Verification items for the finished model (mm, model axes). A direction names the side the tool comes from. Coordinates: 2 decimals unless noted, no trailing zeros. Write each loop counter-clockwise with the first axis right and the second up, starting at its lowest first coordinate (ties: lowest second). Pieces come first, ordered by that corner, then holes. Notation, with made-up numbers: (31.25, 73) -> (44.25, 73) arc R31 ccw to (44.25, 101) -> close; hole circle Ø6 at (87.5, 28). An arc over 180 degrees is marked (long way). Answer in a Markdown table with one row per item.
Autodesk Inventor part; units mm, degrees
ref_plane "Work Plane1" through (1.525, 0, 0) normal (0, 0, 1) x (1, 0, 0)
ref_plane "YZ Plane" through (0, 0, 0) normal (1, 0, 0) x (0, 1, 0)
ref_plane "XZ Plane" through (0, 0, 0) normal (0, 1, 0) x (-1, 0, 0)
sketch "Sketch1" plane through (0, 0, 0) normal (0, 0, 1) x (1, 0, 0)
  line L0 (0, 4) -> (55, 4)
  line L1 (55, 4) -> (55, 0)
  line L2 (55, 0) -> (0, 0)
  line L3 (-11, 0) -> (66, 0)
  line L4 (0, -0.8) -> (0, 4.8)
  line L5 (0, 4) -> (0, 0)
  dimension "d2" = 8
  dimension "d59" = 55
revolve "Body" add sketch "Sketch1" angle 360 about axis through (55, 0, 0) along (-1, 0, 0)
sketch "Sketch2" plane through (0, 0, 0) normal (-1, 0, 0) x (0, 0, 1)
  line L0 (0, 7.5056) -> (6.5, 3.7528)
  line L1 (6.5, 3.7528) -> (6.5, -3.7528)
  line L2 (6.5, -3.7528) -> (0, -7.5056)
  line L3 (0, -7.5056) -> (-6.5, -3.7528)
  line L4 (-6.5, -3.7528) -> (-6.5, 3.7528)
  line L5 (-6.5, 3.7528) -> (0, 7.5056)
  line L6 (-9.1, 0) -> (9.1, 0)
  line L7 (0, 10.5078) -> (0, -10.5078)
  point P0 (0, 0)
  point P1 (0, 0)
  dimension "d11" = 13
extrude "Head" add sketch "Sketch2" along normal blind 5.68
sketch "Sketch4" plane through (0, 0, 0) normal (0, 0, 1) x (1, 0, 0)
  line L0 (-4.9294, 7.8) -> (-5.68, 6.5)
  line L1 (-1.1, 0) -> (-0.234, 0)
  line L2 (-6.7692, 0) -> (0.8552, 0)
  line L3 (-5.68, 7.8) -> (-4.9294, 7.8)
  line L4 (-5.68, 6.5) -> (-5.68, 7.8)
  line L5 (0, 9.36) -> (0, -1.56)
  dimension "d65" = 13
  dimension "d67" = 30
  dimension "d68" = 15.6
  dimension "d69" = 5.68
revolve "Chamfer1" cut sketch "Sketch4" angle 360 about axis through (-1.1, 0, 0) along (1, 0, 0)
thread "Thread"
chamfer "Chamfer2" distance 0.7668 distance2 0.7669 1 edges at (55, -4, 0) measured on face at (55, -1.1806, 1.575)
fillet "Fillet" radius 0.1 1 edges at (0, -4, 0)
ref_plane "Work Plane1" through (1.525, 0, 0) normal (0, 0, 1) x (1, 0, 0)
equation "\"d2\" = GD"
equation "\"d59\" = NLG"
equation "\"d11\" = SW"
equation "\"d3\" = KOH"
equation "\"d15\" = GEL"
equation "\"d6\" = -0.5 * SPD + 0.5 * GD"
equation "\"d71\" = RR"
equation "\"d65\" = SW"
equation "\"d67\" = ANG1"
equation "\"d68\" = 1.2 * SW"
equation "\"d69\" = KOH"
equation "\"NLG\" = 55"
equation "\"GD\" = NND"
equation "\"BDM\" = NND"
equation "\"KOH\" = 5.68"
equation "\"GEL\" = 22"
equation "\"SW\" = 13"
equation "\"SW0\" = SW"
equation "\"SPD\" = NND - 1.2269 * PTC"
equation "\"SD2\" = NND"
equation "\"SD\" = 0"
equation "\"ANG1\" = 30deg"
equation "\"GAL\" = 0.61345 * PTC"
equation "\"GUL\" = 0.61345 * PTC"
equation "\"RR\" = 0.1"
equation "\"RR1\" = 0.4"
equation "\"GD1\" = THREADDIA - 1.2269 * PTC"
equation "\"THREADDIA\" = 8"
equation "\"TOA\" = 30deg"
equation "\"PTC\" = 1.25"
equation "\"KOH1\" = 3.7"
equation "\"NND\" = 8"
equation "\"E0\" = 1.155 * SW"
properties part number "ANSI B18.2.3.5M - M8 x 1.25 x 55" material "Steel, Mild"
1. Thickness scan on line 1 (X direction, y = 3.5, z = 5); line 2 (Y direction, x = -2.5, z = 1.75); line 3 (Z direction, x = 50.5, y = 0.25). Record the ranges inside material, lowest first. Write a range as from..to.
Geometry says:
| item | result |
|---|---|
| line 1 | -5.68..0 |
| line 2 | -6.5..6.5 |
| line 3 | -3.99..3.99 |
2. Tool access check on faces 1 (the flat face through (0, -3.2, 2.8)), 2 (the flat face through (55, 0, 0)). Record the directions out of +Z, -Z, +X, -X, +Y, -Y that give a thin tool (end or side, any length) a straight path to the whole face; none if there is none.
Geometry says:
| item | result |
|---|---|
| face 1 | +X |
| face 2 | +Z, -Z, +X, +Y, -Y |
3. Section check A-A, the plane x = -1.5. Record the boundary of the cut face in (y, z), plus the area to 3 significant figures.
Geometry says:
| item | result |
|---|---|
| outline | (-7.51, 0) -> (-3.75, -6.5) -> (3.75, -6.5) -> (7.51, 0) -> (3.75, 6.5) -> (-3.75, 6.5) -> close |
| area | 146 mm^2 |
4. Depth check by flat-ended pin: P1, Ø3, axis at x = 31, y = 3.5, coming from the -Z side; P2, Ø8, axis at x = 19, y = -1.5, coming from the +Z side. Enter the tip coordinate at first touch or a pass-through.
Geometry says:
| item | result |
|---|---|
| P1 | z = -3.46 |
| P2 | z = 4 |
